from build123d import *

# Parameters (mm, degrees)
SKETCH_1_W          = 40
SKETCH_1_H          = 65
EXTRUDE_1_DEPTH     = 9
CHAMFER_1_SIZE      = 2
FILLET_3_R          = 20
SKETCH_2_W          = 21
SKETCH_2_H          = 41
CUT_EXTRUDE_1_DEPTH = 10
SKETCH_3_W          = 2
SKETCH_3_H          = 5.5
CUT_EXTRUDE_2_DEPTH = 10
SKETCH_4_R          = 1.5
CUT_EXTRUDE_3_DEPTH = 10
SKETCH_5_R          = 1.5
CUT_EXTRUDE_4_DEPTH = 10
FILLET_4_R          = 1
CUT_EXTRUDE_5_DEPTH = 3.2
CHAMFER_2_SIZE      = 0.5


with BuildPart() as part:
    # 草图1 → 凸台-拉伸1 (new body)
    with BuildSketch(Plane.XY):
        with Locations((20, -37.5)):
            Rectangle(SKETCH_1_W, SKETCH_1_H)
    extrude(amount=EXTRUDE_1_DEPTH)

    # 倒角1
    chamfer_1_edges = [part.edges().sort_by_distance(p)[0] for p in [
        (0, -5, 4.5),
        (40, -5, 4.5),
    ]]
    chamfer(chamfer_1_edges, length=CHAMFER_1_SIZE)

    # 圆角3
    fillet_3_edges = [part.edges().sort_by_distance(p)[0] for p in [
        (0, -70, 4.5),
        (40, -70, 4.5),
    ]]
    fillet(fillet_3_edges, radius=FILLET_3_R - 0.0001)  # a hair under: the kernel refuses the full size

    # 草图2 → 切除-拉伸1 (cut)
    with BuildSketch(Plane(origin=(0, 0, 0), x_dir=(-1, 0, 0), z_dir=(0, 0, -1))):
        with Locations((-20, -40.32)):
            Rectangle(SKETCH_2_W, SKETCH_2_H)
    extrude(amount=-CUT_EXTRUDE_1_DEPTH, mode=Mode.SUBTRACT)

    # 草图3 → 切除-拉伸2 (cut)
    with BuildSketch(Plane.XY.offset(9)):
        with Locations((20, -17.07)):
            Rectangle(SKETCH_3_W, SKETCH_3_H)
        with Locations((20, -63.57)):
            Rectangle(SKETCH_3_W, SKETCH_3_H)
    extrude(amount=-CUT_EXTRUDE_2_DEPTH, mode=Mode.SUBTRACT)

    # 草图4 → 切除-拉伸3 (cut)
    with BuildSketch(Plane(origin=(0, 0, 0), x_dir=(-1, 0, 0), z_dir=(0, 0, -1))):
        with Locations((-25, -16.07)):
            Circle(SKETCH_4_R)
        with Locations((-15, -16.07)):
            Circle(SKETCH_4_R)
        with Locations((-25, -64.57)):
            Circle(SKETCH_4_R)
        with Locations((-15, -64.57)):
            Circle(SKETCH_4_R)
    extrude(amount=-CUT_EXTRUDE_3_DEPTH, mode=Mode.SUBTRACT)

    # 草图5 → 切除-拉伸4 (cut)
    with BuildSketch(Plane(origin=(0, 0, 0), x_dir=(-1, 0, 0), z_dir=(0, 0, -1))):
        with Locations((-32, -9)):
            Circle(SKETCH_5_R)
        with Locations((-20, -9)):
            Circle(SKETCH_5_R)
        with Locations((-8, -9)):
            Circle(SKETCH_5_R)
    extrude(amount=-CUT_EXTRUDE_4_DEPTH, mode=Mode.SUBTRACT)

    # 圆角4
    fillet_4_edges = [part.edges().sort_by_distance(p)[0] for p in [
        (21, -66.32, 4.5),
        (19, -66.32, 4.5),
        (21, -14.32, 4.5),
        (19, -14.32, 4.5),
    ]]
    fillet(fillet_4_edges, radius=FILLET_4_R - 0.0001)  # a hair under: the kernel refuses the full size

    # 草图7 → 切除-拉伸5 (cut)
    with BuildSketch(Plane(origin=(0, 0, 0), x_dir=(-1, 0, 0), z_dir=(0, 0, -1))):
        with BuildLine():
            Line((-34.9, -9), (-34.9, -5))
            Line((-34.9, -5), (-29.1, -5))
            Line((-29.1, -5), (-29.1, -9))
            ThreePointArc((-29.1, -9), (-32, -11.9), (-34.9, -9))
        make_face()
        with BuildLine():
            Line((-17.1, -9), (-17.1, -5))
            Line((-17.1, -5), (-22.9, -5))
            Line((-22.9, -5), (-22.9, -9))
            ThreePointArc((-22.9, -9), (-20, -11.9), (-17.1, -9))
        make_face()
        with BuildLine():
            Line((-5.1, -9), (-5.1, -5))
            Line((-5.1, -5), (-10.9, -5))
            Line((-10.9, -5), (-10.9, -9))
            ThreePointArc((-10.9, -9), (-8, -11.9), (-5.1, -9))
        make_face()
    extrude(amount=-CUT_EXTRUDE_5_DEPTH, mode=Mode.SUBTRACT)

    # 倒角2
    chamfer_2_edges = [part.edges().sort_by_distance(p)[0] for p in [
        (16.5, -16.07, 0),
        (26.5, -64.57, 0),
        (16.5, -64.57, 0),
        (26.5, -16.07, 0),
        (32, -11.9, 0),
        (29.1, -7, 0),
        (34.9, -7, 0),
        (20, -11.9, 0),
        (17.1, -7, 0),
        (22.9, -7, 0),
        (8, -11.9, 0),
        (5.1, -7, 0),
        (10.9, -7, 0),
    ]]
    chamfer(chamfer_2_edges, length=CHAMFER_2_SIZE)


solid = part.part
For this review, take the finished solid that the model builds, in its own axes (mm). A direction names the side the tool comes from. Round coordinates to 2 decimals unless told otherwise and drop trailing zeros. Loops run counter-clockwise (first coordinate to the right, second up) from the corner with the lowest first, then second, coordinate; pieces in that order, holes last. Notation, with made-up numbers: (75.25, 67) - (110.25, 67) arc R21 cw to (110.25, 72) - close; hole circle Ø7 at (42.25, 84). An arc over 180 degrees is marked (long way). Answer as CSV lines item,"result".
(1) Consider section B-B on z = 6.25. Give the number of separate pieces and of enclosed holes in the cut face, then the cut area to 3 significant figures.
Checked values:
separate pieces,"1"
enclosed holes,"8"
area,"1,490 mm2"
(2) Mouldability with a two-part tool opening along X and no side actions: class faces 4 (the face through (1, -6, 4)), 5 (the face through (21, -63, 5)), 6 (the face through (33.986, -64.297, 4.563)) as +X half, -X half, draft (parallel to the pull), parting line (faces both ways), or undercut.
Checked values:
face 4,"-X half"
face 5,"undercut"
face 6,"+X half"
(3) Tool access review of faces 1 (the face through (40, -29, 4)), 2 (the face through (20, -7, 3.2)), 3 (the face through (14, -19.82, 4)): name each direction out of +Z, -Z, +X, -X, +Y, -Y from which nothing blocks a thin tool from reaching the whole face with its end or side.
Checked values:
face 1,"+Z, -Z, +X, +Y, -Y"
face 2,"-Z, +Y"
face 3,"+Z, -Z"
(4) Consider section A-A on y = -16.07. Give the boundary of the cut face in (x, z).
Checked values:
outline,"(0, 0) - (13, 0) - (13.5, 0.5) - (13.5, 9) - (0, 9) - close; (16.5, 0.5) - (17, 0) - (19, 0) - (19, 9) - (16.5, 9) - close; (21, 0) - (23, 0) - (23.5, 0.5) - (23.5, 9) - (21, 9) - close; (26.5, 0.5) - (27, 0) - (40, 0) - (40, 9) - (26.5, 9) - close"
(5) Consider section C-C on y = -35. Give the boundary of the cut face in (x, z), then the cut area to 3 significant figures.
Checked values:
outline,"(0, 0) - (9.5, 0) - (9.5, 9) - (0, 9) - close; (30.5, 0) - (40, 0) - (40, 9) - (30.5, 9) - close"
area,"171 mm2"
(6) Wall thickness on line 1 (X direction, y = -19, z = 4.25); line 2 (X direction, y = -48, z = 2.25); line 3 (X direction, y = -8.5, z = 7.75): over which ranges is each line inside the solid? List them lowest first.
Checked values:
line 1,"x = 0 to 19, 21 to 40"
line 2,"x = 0 to 9.5, 30.5 to 40"
line 3,"x = 0 to 6.59, 9.41 to 18.59, 21.41 to 30.59, 33.41 to 40"
(7) Insertion check: P1, Ø0.8, axis at y = -6.5, z = 2.5, coming from the +X side; P2, Ø1.5, axis at y = -60.5, z = 8, coming from the -X side; P3, Ø1.7, axis at x = 7, y = -7.5, coming from the -Z side. Each pin has a flat end and moves straight along its axis. Give the tip position at first contact, or say it passes through.
Checked values:
P1,"stops at x = 39.9"
P2,"stops at x = 2.54"
P3,"stops at z = 3.2"
